The listing builds one solid part. Answer for the finished solid, in the listing's coordinates (mm). A direction names the side the tool comes from. Coordinates: 2 decimals unless noted, no trailing zeros. Loops run counter-clockwise (first coordinate to the right, second up) from the corner with the lowest first, then second, coordinate; pieces in that order, holes last. Notation, with made-up numbers: M 8.25,23 L 14.25,23 A28 cw 14.25,61 Z; hole C 48.5,-20.75 d7. An arc over 180 degrees is marked long. Answer as a JSON object with one key per item and string values. Group by question number.
1. A cutting plane is placed at C-C on z = -0.75. Give the vertices of the cut face in (x, y), and give its area (3 significant figures).
2. Given pin 1 (3.5 mm diameter, centred on y = 7.5, z = 1, fed in from -X); pin 2 (4 mm diameter, centred on x = -7.34, y = 7.48, fed in from -Z); pin 3 (1.5 mm diameter, centred on y = 6, z = 1.5, fed in from +X), each flat-ended and moving along its own axis, determine where each tip first touches the part or whether it passes through.
3. For faces 1 (the face through (-10, 7, 4)), 2 (the face through (-4.3, 7, 1)), 3 (the face through (4.3, 7, 1)), determine the directions among +Z, -Z, +X, -X, +Y, -Y from which every point of the face is accessible in a straight line to the end or side of a thin tool.
4. Determine the mould class of faces 4 (the face through (2.024, 7.138, 1.29)), 5 (the face through (10, 7, 4)), 6 (the face through (0, 7, 4.323)), 7 (the face through (-7.2, 5.5, 2.823)) for opening direction Z: released by +Z, released by -Z, zero draft, split by the parting line, or undercut.
5. A cutting plane is placed at B-B on x = 0. Give the vertices of the cut face in (y, z), and give its area (3 significant figures).
6. A cutting plane is placed at A-A on y = 8.75. State how many separate pieces and enclosed holes the cut face has, and give its area (3 significant figures).
7. Straight lines are drawn through the part: L1, parallel to X at y = 13.75, z = 1.25; L2, parallel to Z at x = 6, y = 5.25; L3, parallel to X at y = 11, z = 1. For each, find the intervals that lie inside material, in ascending order.
from build123d import *

# Parameters (mm, degrees)
SKETCH1_R           = 4.3
SKETCH1_R_2         = 2.4
SKETCH1_W           = 20
SKETCH1_H           = 1.5
BOSS_EXTRUDE1_DEPTH = 14.478
SKETCH2_W           = 1.056255113
SKETCH2_H           = 14.478
BOSS_EXTRUDE2_DEPTH = 3
SKETCH3_W           = 1.056255113
SKETCH3_H           = 14.478
BOSS_EXTRUDE3_DEPTH = 3
SKETCH4_R           = 1.651
CUT_EXTRUDE1_DEPTH  = 3


with BuildPart() as part:
    # Sketch1 → Boss-Extrude1 (new body)
    # profile 1 of 2: a face of its own
    with BuildSketch(Plane(origin=(0, 0, 0), x_dir=(1, 0, 0), z_dir=(0, 1, 0))):
        Circle(SKETCH1_R)
        with Locations(Location((0, 0, 0), (0, 0, 270))):
            Circle(SKETCH1_R_2, mode=Mode.SUBTRACT)
    # profile 2 of 2: a face of its own
    with BuildSketch(Plane(origin=(0, 0, 0), x_dir=(1, 0, 0), z_dir=(0, 1, 0))):
        with Locations((0, -3.572785701)):
            Rectangle(SKETCH1_W, SKETCH1_H)
    extrude(amount=BOSS_EXTRUDE1_DEPTH)

    # Sketch2 → Boss-Extrude2 (add)
    with BuildSketch(Plane(origin=(0, 0, 2.822785701), x_dir=(-1, 0, 0), z_dir=(0, 0, -1))):
        with Locations((-3.771872444, 7.239)):
            Rectangle(SKETCH2_W, SKETCH2_H)
    extrude(amount=BOSS_EXTRUDE2_DEPTH)

    # Sketch3 → Boss-Extrude3 (add)
    with BuildSketch(Plane(origin=(0, 0, 2.822785701), x_dir=(-1, 0, 0), z_dir=(0, 0, -1))):
        with Locations((3.771872444, 7.239)):
            Rectangle(SKETCH3_W, SKETCH3_H)
    extrude(amount=BOSS_EXTRUDE3_DEPTH)

    # Sketch4 → Cut-Extrude1 (cut)
    with BuildSketch(Plane(origin=(0, 0, 2.822785701), x_dir=(-1, 0, 0), z_dir=(0, 0, -1))):
        with Locations((-7.335568172, 7.478)):
            Circle(SKETCH4_R)
        with Locations((7.335568172, 7.478)):
            Circle(SKETCH4_R)
    extrude(amount=-CUT_EXTRUDE1_DEPTH, mode=Mode.SUBTRACT)


solid = part.part
From the geometry:
{
 "1": {"outline": "M -4.23,0 L -2.28,0 L -2.28,14.48 L -4.23,14.48 Z; M 2.28,0 L 4.23,0 L 4.23,14.48 L 2.28,14.48 Z", "area": "56.6 mm²"},
 "2": {"pin 1": "stops at x = -4.3", "pin 2": "stops at z = 2.82", "pin 3": "stops at x = 4.3"},
 "3": {"face 1": "+Z, -Z, -X, +Y, -Y", "face 2": "-Z, -X, +Y, -Y", "face 3": "-Z, +X, +Y, -Y"},
 "4": {"face 4": "undercut", "face 5": "zero draft", "face 6": "released by +Z", "face 7": "released by -Z"},
 "5": {"outline": "M 0,-4.3 L 14.48,-4.3 L 14.48,-2.4 L 0,-2.4 Z; M 0,2.4 L 14.48,2.4 L 14.48,4.32 L 0,4.32 Z", "area": "55.3 mm²"},
 "6": {"separate pieces": "3", "enclosed holes": "1", "area": "58.9 mm²"},
 "7": {"L1": "x = -4.3 to -2.05, 2.05 to 4.3", "L2": "z = 2.82 to 4.32", "L3": "x = -4.3 to -2.18, 2.18 to 4.3"}
}
